Input: part model. Units: mm. Frame: model coordinates. Round coordinates to 2 decimals unless told otherwise and drop trailing zeros. Loops run counter-clockwise (first coordinate to the right, second up) from the corner with the lowest first, then second, coordinate; pieces in that order, holes last. Notation, with made-up numbers: M 17,81.5 L 48,81.5 A24 cw 48,116.5 Z; hole C -22,27 d9. An arc over 180 degrees is marked long. Return JSON: item names as keys, results as strings. Group by question number.
1) Material intervals for line 1 (Z direction, x = -25, y = -13.25); line 2 (Z direction, x = -4, y = -5.25); line 3 (X direction, y = -18.5, z = 26), sorted ascending. Write a range as from..to.
2) Section B-B (z = 0). Output: boundary loops of the cut face in (x, y), plus the area to 3 significant figures.
3) Section A-A (x = 0). Output: boundary loops of the cut face in (y, z).
4) Mould query, pull axis Z, two halves, no side actions, for faces 1 (the face through (32.493, -10.14, -0.33)), 2 (the face through (52, -10, -29)), 3 (the face through (-52, -1, 0)), 4 (the face through (-52, -10, 29)). Classes: +Z half, -Z half, draft (parallel to the pull), parting line (faces both ways), or undercut.
5) Contact query for a flat-ended pin moving along its axis: P1, Ø9, axis at x = 25, z = 0, coming from the +Y side. Output: stop coordinate, or through.
6) Section D-D (x = 24.5). Output: boundary loops of the cut face in (y, z).
7) Section C-C (y = -13.5). Output: boundary loops of the cut face in (x, z).
from build123d import *

# Parameters (mm, degrees)
F0_W     = 105
F0_H     = 60
F1_DEPTH = 20
F2_R     = 7.5
F3_DEPTH = 25
F4_R     = 2.5


with BuildPart() as f1:
    # F0 (on Front) → F1 (new body)
    with BuildSketch(Plane.XZ):
        Rectangle(F0_W, F0_H)
    extrude(amount=F1_DEPTH)

    # F2 (on face) → F3 (cut)
    with BuildSketch(Plane.XZ.offset(20)):
        with BuildLine():
            ThreePointArc((-7.5, 0), (0, -7.5), (7.5, 0))
            ThreePointArc((7.5, 0), (0, 7.5), (-7.5, 0))
        make_face()
        with Locations((-25, 0)):
            Circle(F2_R)
        with BuildLine():
            ThreePointArc((32.5, 0), (25, 7.5), (17.5, 0))
            ThreePointArc((17.5, 0), (25, -7.5), (32.5, 0))
        make_face()
    extrude(amount=-F3_DEPTH, mode=Mode.SUBTRACT)

    # F4
    f4_edges = [f1.edges().sort_by_distance(p)[0] for p in [
        (52.5, -10, -30),
        (52.5, -10, 30),
        (52.5, 0, 0),
        (52.5, -20, 0),
        (-52.5, -10, 30),
        (0, 0, 30),
        (0, -20, 30),
        (-52.5, -10, -30),
        (-52.5, 0, 0),
        (-52.5, -20, 0),
        (0, 0, -30),
        (0, -20, -30),
    ]]
    fillet(f4_edges, radius=F4_R)


solid = f1.part
Returned:
{
 "1": {"line 1": "z = -30..-7.5, 7.5..30", "line 2": "z = -30..-6.34, 6.34..30", "line 3": "x = -52.29..52.29"},
 "2": {"outline": "M -52.5,-17.5 A2.5 ccw -50,-20 L -32.5,-20 L -32.5,0 L -50,0 A2.5 ccw -52.5,-2.5 Z; M -17.5,-20 L -7.5,-20 L -7.5,0 L -17.5,0 Z; M 7.5,-20 L 17.5,-20 L 17.5,0 L 7.5,0 Z; M 32.5,-20 L 50,-20 A2.5 ccw 52.5,-17.5 L 52.5,-2.5 A2.5 ccw 50,0 L 32.5,0 Z", "area": "1,190 mm^2"},
 "3": {"outline": "M -20,-27.5 A2.5 ccw -17.5,-30 L -2.5,-30 A2.5 ccw 0,-27.5 L 0,-7.5 L -20,-7.5 Z; M -20,7.5 L 0,7.5 L 0,27.5 A2.5 ccw -2.5,30 L -17.5,30 A2.5 ccw -20,27.5 Z"},
 "4": {"face 1": "undercut", "face 2": "-Z half", "face 3": "draft", "face 4": "+Z half"},
 "5": {"P1": "passes through"},
 "6": {"outline": "M -20,-27.5 A2.5 ccw -17.5,-30 L -2.5,-30 A2.5 ccw 0,-27.5 L 0,-7.48 L -20,-7.48 Z; M -20,7.48 L 0,7.48 L 0,27.5 A2.5 ccw -2.5,30 L -17.5,30 A2.5 ccw -20,27.5 Z"},
 "7": {"outline": "M -52.5,-27.5 A2.5 ccw -50,-30 L 50,-30 A2.5 ccw 52.5,-27.5 L 52.5,27.5 A2.5 ccw 50,30 L -50,30 A2.5 ccw -52.5,27.5 Z; hole C -25,0 d15; hole C 0,0 d15; hole C 25,0 d15"}
}
